The drawing under review shows one solid part. Ordinate dimensions are in mm from its lowest x, y, z. A direction names the side the tool comes from. Coordinates: 2 decimals unless noted, no trailing zeros. Order: outer loops, then holes, each group sorted by start corner. A loop starts at its lowest first (then second) coordinate and runs counter-clockwise, first axis right, second up. Notation, with made-up numbers: (-1, -13) -> (23, -13) arc R19 ccw to (23, 7) -> close; hole circle Ø4 at (21, 65.5). An arc over 180 degrees is marked (long way). Put each result on its own line as item: value.
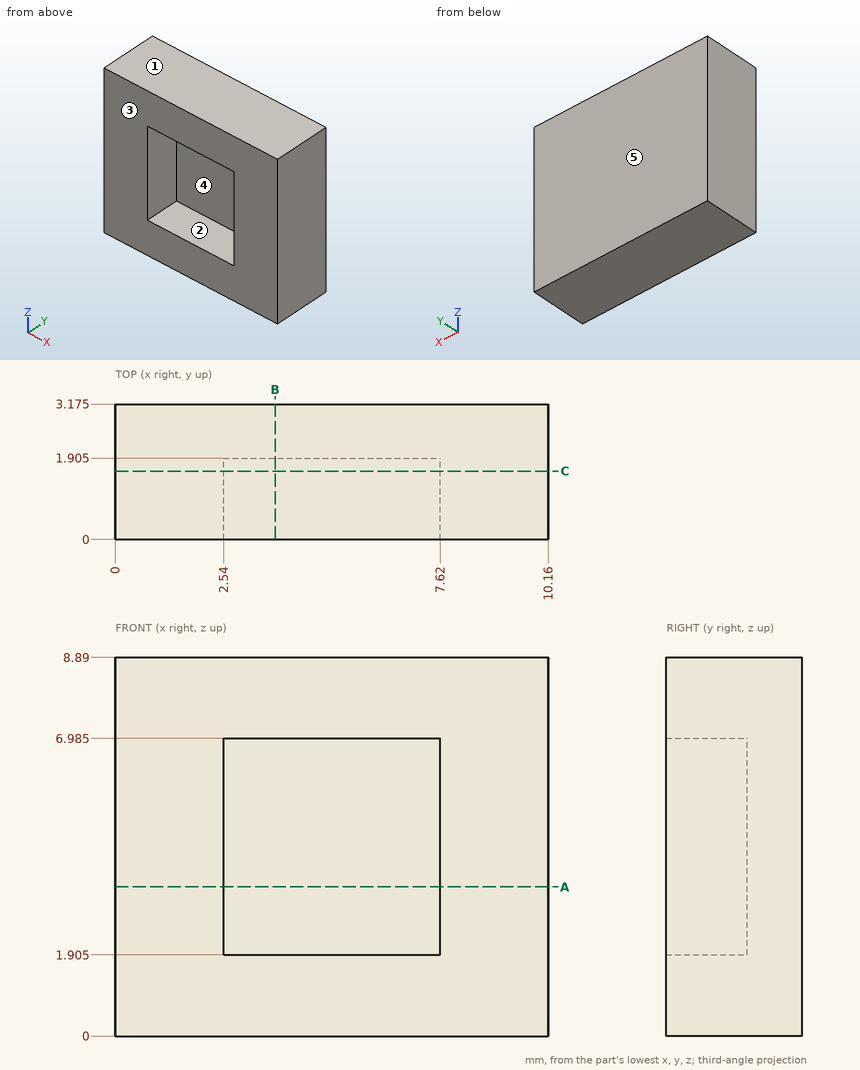
Item 1: Consider section C-C on y = 1.6. Write out the cut boundary in (x, z) (3 decimals), and give its area (3 significant figures).
Answers below:
outline: (0, 0) -> (10.16, 0) -> (10.16, 8.89) -> (0, 8.89) -> close; hole (2.54, 1.905) -> (7.62, 1.905) -> (7.62, 6.985) -> (2.54, 6.985) -> close
area: 64.5 mm^2
Item 2: For pin 1 Ø1 at (x, y) = (4, 0.5) entering from -Z, flat-tipped, find the tip position at first contact; note if it passes through.
Answers below:
pin 1: z = 0
Item 3: Consider section B-B on x = 3.75. Write out the cut boundary in (y, z) (3 decimals), and give its area (3 significant figures).
Answers below:
outline: (0, 0) -> (3.175, 0) -> (3.175, 8.89) -> (0, 8.89) -> (0, 6.985) -> (1.905, 6.985) -> (1.905, 1.905) -> (0, 1.905) -> close
area: 18.5 mm^2
Item 4: For line 1 (X direction, y = 1.25, z = 5.25); line 2 (Z direction, x = 4.5, y = 0.6) (3 decimals); line 3 (Y direction, x = 3.5, z = 3.25) (3 decimals), list the stretches that pass through material, from the lowest coordinate up. Write a range as from..to.
Answers below:
line 1: 0..2.54, 7.62..10.16
line 2: 0..1.905, 6.985..8.89
line 3: 1.905..3.175
Item 5: For the marked faces 4 and 5, list the 3-axis set-ups (+Z, -Z, +X, -X, +Y, -Y) from which the entire face can be reached by the end or side of a thin tool; tool diameter is ignored.
Answers below:
face 4: -Y
face 5: +Z, -Z, +X, -X, +Y
Item 6: Mouldability with a two-part tool opening along Z and no side actions: class the marked faces 1, 2 and 3 as +Z half, -Z half, draft (parallel to the pull), parting line (faces both ways), or undercut.
Answers below:
face 1: +Z half
face 2: undercut
face 3: draft
Item 7: Consider section A-A on z = 3.5. Write out the cut boundary in (x, y) (3 decimals), and give its area (3 significant figures).
Answers below:
outline: (0, 0) -> (2.54, 0) -> (2.54, 1.905) -> (7.62, 1.905) -> (7.62, 0) -> (10.16, 0) -> (10.16, 3.175) -> (0, 3.175) -> close
area: 22.6 mm^2
